```python
from build123d import *

# Parameters (mm, degrees)
SKETCH1_W                   = 152.4
SKETCH1_H                   = 25.4
EXTRUDE1_DEPTH              = 6.35
SKETCH2_W                   = 25.4
SKETCH2_H                   = 133.35
EXTRUDE2_DEPTH              = 6.35
SKETCH3_W                   = 57.15
SKETCH3_H                   = 50.8
EXTRUDE3_DEPTH              = 6.35
CHAMFER1_SIZE               = 2.54
CHAMFER1_SIZE2              = 6.978592645
F_3_8_CLEARANCE_HOLE1_D     = 10.0838
F_3_8_CLEARANCE_HOLE1_DEPTH = 38.1
F_3_8_CLEARANCE_HOLE1_TIP   = 3.029479155


with BuildPart() as part:
    # Sketch1 → Extrude1 (new body)
    with BuildSketch(Plane.XY):
        Rectangle(SKETCH1_W, SKETCH1_H)
    extrude(amount=EXTRUDE1_DEPTH)

    # Sketch2 → Extrude2 (add)
    with BuildSketch(Plane.XY.offset(6.35)):
        with Locations((34.29, 53.975)):
            Rectangle(SKETCH2_W, SKETCH2_H)
    extrude(amount=EXTRUDE2_DEPTH)

    # Sketch3 → Extrude3 (add)
    with BuildSketch(Plane(origin=(0, 0, 6.35), x_dir=(-1, 0, 0), z_dir=(0, 0, -1))):
        with Locations((-50.165, 95.25)):
            Rectangle(SKETCH3_W, SKETCH3_H)
    extrude(amount=EXTRUDE3_DEPTH)

    # Chamfer1
    chamfer1_edges = [part.edges().sort_by_distance(p)[0] for p in [
        (78.74, 69.85, 3.175),
    ]]
    chamfer1_side = [part.faces().sort_by_distance(p)[0] for p in [
        (78.74, 95.25, 3.175),
    ]]
    chamfer(chamfer1_edges, length=CHAMFER1_SIZE, length2=CHAMFER1_SIZE2, reference=chamfer1_side[0])

    # 3/8 Clearance Hole1
    with Locations(Plane(origin=(63.5, 0, 6.35), x_dir=(1, 0, 0), z_dir=(0, 0, 1))):
        with Locations((0, 0)):
            Hole(F_3_8_CLEARANCE_HOLE1_D / 2, depth=F_3_8_CLEARANCE_HOLE1_DEPTH)
            with Locations((0, 0, -(F_3_8_CLEARANCE_HOLE1_DEPTH + F_3_8_CLEARANCE_HOLE1_TIP / 2))):  # 118° drill point
                Cone(0, F_3_8_CLEARANCE_HOLE1_D / 2, F_3_8_CLEARANCE_HOLE1_TIP, mode=Mode.SUBTRACT)


solid = part.part
```
Geometry: final body of the model. Coordinates: model frame, mm. A direction names the side the tool comes from. Coordinates: 2 decimals unless noted, no trailing zeros. Write each loop counter-clockwise with the first axis right and the second up, starting at its lowest first coordinate (ties: lowest second). Pieces come first, ordered by that corner, then holes. Notation, with made-up numbers: M 19.25,-16.75 L 28.25,-16.75 A18 cw 28.25,-10.75 Z; hole C -17.5,41.5 d8. An arc over 180 degrees is marked long. Use CSV: the item, a comma, the result in double quotes. Start each with the question number.
1. Cut plane C-C on z = 9.75. Return the cut outline in (x, y), plus the area to 3 significant figures.
2. Cut plane A-A on x = 63.5. Return the cut outline in (y, z), plus the area to 3 significant figures.
3. First-contact query: P1, Ø12.5, axis at x = -8.5, y = 2.5, coming from the +Z side; P2, Ø3, axis at x = -12.5, z = 2.5, coming from the +Y side; P3, Ø3, axis at y = 4, z = 1.5, coming from the +X side. Flat tips, straight axial feed; report the tip coordinate or a pass-through.
4. Cut plane D-D on y = 44. Return the cut outline in (x, z), plus the area to 3 significant figures.
5. Mould query, pull axis Y, two halves, no side actions, for faces 5 (the face through (44, 120.65, 5)), 6 (the face through (-1, -12.7, 3)), 7 (the face through (34, 42, 6.35)), 8 (the face through (58, 0, 6.35)). Classes: pulls with the +Y half, pulls with the -Y half, needs draft (parallel to the pull), parting line crosses it, or undercut.
6. Cut plane B-B on y = 0. Return the cut outline in (x, z), plus the area to 4 significant figures.
7. Ray query, probe 1 along Y at (x, z) = (63.5, 3); probe 2 along Y at (x, z) = (43.5, 2.25); probe 3 along Z at (x, y) = (30.5, 52.5). Return the intervals inside material, ascending.
8. Reachability of faces 1 (the face through (76.2, 0, 3)), 2 (the face through (-28, 0, 6.35)), 3 (the face through (47, 69.85, 3)), 4 (the face through (46.99, 53, 9)) from +Z, -Z, +X, -X, +Y, -Y: full face, straight path, thin tool, end or side. Return the list, or none.
Entries:
1,outline,"M 21.59,-12.7 L 46.99,-12.7 L 46.99,120.65 L 21.59,120.65 Z"
1,area,"3,390 mm²"
2,outline,"M -12.7,0 L -5.04,0 L -5.04,6.35 L -12.7,6.35 Z; M 5.04,0 L 12.7,0 L 12.7,6.35 L 5.04,6.35 Z; M 69.85,0 L 120.65,0 L 120.65,6.35 L 69.85,6.35 Z"
2,area,"420 mm²"
3,P1,"z = 6.35"
3,P2,"y = 12.7"
3,P3,"x = 76.2"
4,outline,"M 21.59,6.35 L 46.99,6.35 L 46.99,12.7 L 21.59,12.7 Z"
4,area,"161 mm²"
5,face 5,"pulls with the +Y half"
5,face 6,"pulls with the -Y half"
5,face 7,"undercut"
5,face 8,"needs draft"
6,outline,"M -76.2,0 L 58.46,0 L 58.46,6.35 L 46.99,6.35 L 46.99,12.7 L 21.59,12.7 L 21.59,6.35 L -76.2,6.35 Z; M 68.54,0 L 76.2,0 L 76.2,6.35 L 68.54,6.35 Z"
6,area,"1,065 mm²"
7,probe 1,"-12.7 to -5.04, 5.04 to 12.7, 69.85 to 120.65"
7,probe 2,"-12.7 to 12.7, 69.85 to 120.65"
7,probe 3,"6.35 to 12.7"
8,face 1,"+Z, -Z, +X, -Y"
8,face 2,"+Z, -X, +Y, -Y"
8,face 3,"-Z, +X, -X"
8,face 4,"+Z, +X, +Y, -Y"
